Autodesk Inventor part; units mm, degrees
ref_plane "YZ Plane" through (0, 0, 0) normal (1, 0, 0) x (0, 1, 0)
ref_plane "XZ Plane" through (0, 0, 0) normal (0, 1, 0) x (-1, 0, 0)
ref_plane "XY Plane" through (0, 0, 0) normal (0, 0, 1) x (1, 0, 0)
sketch "Sketch1" plane through (0, 0, 0) normal (0, 1, 0) x (-1, 0, 0)
  arc A0 (3.2, -5.2536) -> (17, 0) centre (9.1, 0) ccw
  line L0 (3.2, -5.2536) -> (3.2, -15)
  line L1 (3.2, -15) -> (0, -15)
  line L2 (0, -15) -> (0, 15)
  line L3 (0, 15) -> (3.2, 15)
  line L4 (3.2, 15) -> (3.2, 5.2536)
  arc A1 (17, 0) -> (3.2, 5.2536) centre (9.1, 0) ccw
  line L5 (9.1, 7.9) -> (9.1, -7.9) construction
  line L6 (3.2, 5.2536) -> (17, 0) construction
  line L7 (3.2, -5.2536) -> (17, 0) construction
  point P0 (0, 0)
  point P1 (0, 0)
  dimension "d0" = 3.2
  dimension "d1" = 30
  dimension "d5" = 15.8
  dimension "d6" = 17
extrude "Extrusion1" add sketch "Sketch1" along normal blind 51
sketch "Sketch2" plane through (0, 0, 15) normal (1, 0, 0) x (0, 0, -1)
  circle A0 centre (25.7, 45.35) radius 1.65
  circle A1 centre (4.3, 5.65) radius 1.65
  line L0 (25.7, 45.35) -> (25.7, 5.65) construction
  line L1 (25.7, 5.65) -> (4.3, 5.65) construction
  line L2 (30, 0) -> (30, 51)
  line L3 (0, 0) -> (0, 51)
  line L4 (25.7, 45.35) -> (30, 45.35) construction
  line L5 (25.7, 45.35) -> (30, 51) construction
  line L6 (0, 0) -> (4.3, 5.65) construction
  line L7 (4.3, 5.65) -> (0, 5.65) construction
  line L8 (30, 39.7) -> (22.9, 39.7)
  line L9 (22.9, 39.7) -> (22.9, 0)
  line L10 (22.9, 0) -> (30, 0)
  line L11 (0, 11.3) -> (7.1, 11.3)
  line L12 (7.1, 11.3) -> (7.1, 51)
  line L13 (7.1, 51) -> (0, 51)
  line L14 (25.7, 45.35) -> (30, 39.7) construction
  point P0 (15, 0)
  dimension "d9" = 21.4
  dimension "d10" = 39.7
  dimension "d11" = 3.3
  dimension "d12" = 2.8
extrude "Extrusion2" cut sketch "Sketch2" against normal up to surface (3.2 mm away)
sketch "Sketch3" plane through (0, 0, 0) normal (0, -1, 0) x (1, 0, 0)
  arc A0 (-3.2, 5.2536) -> (-3.2, -5.2536) centre (-9.1, 0) ccw
  circle A1 centre (-9.1, 0) radius 1.5875
  point P0 (0, 0)
  dimension "d15" = 3.175
extrude "Extrusion3" add sketch "Sketch3" along normal blind 11
sketch "Sketch4" plane through (0, 51, 0) normal (0, 1, 0) x (1, 0, 0)
  arc A0 (-3.2, 5.2536) -> (-3.2, -5.2536) centre (-9.1, 0) ccw construction
  circle A1 centre (-9.1, 0) radius 1.5875
  point P0 (0, 0)
  dimension "d18" = 3.175
extrude "Extrusion4" add sketch "Sketch4" along normal blind 11
properties part number "Power Resistor - HSA50" material "Gold"
Could you check a few things on this model? Use its own coordinates, in mm. A direction names the side the tool comes from. Give positions to 0.01 mm unless a question says otherwise; leave off trailing zeros. Loops run counter-clockwise (first coordinate to the right, second up) from the corner with the lowest first, then second, coordinate; pieces in that order, holes last. Notation, with made-up numbers: (14.5, 69.5) -> (68.5, 69.5) arc R17 cw to (68.5, 89.5) -> close; hole circle Ø11 at (-31.75, 71.5). An arc over 180 degrees is marked (long way). Put each result on its own line as item: value.
(1) Please list where these lines run through material, in increasing order: probe 1 along Y at (x, z) = (-2.5, 10.7); probe 2 along Y at (x, z) = (-2.4, -10.7); probe 3 along X at (y, z) = (31.5, -6.5). Write a range as [from, to].
Computed:
probe 1: [0, 4], [7.3, 11.3]
probe 2: [39.7, 43.7], [47, 51]
probe 3: [-13.59, -4.61], [-3.2, 0]
(2) Imagine slicing it at A-A on y = 5.65. Write out the boundary of the cut face in (x, z), plus the area to 3 significant figures.
Computed:
outline: (-17, 0) arc R7.9 ccw to (-3.2, -5.25) -> (-3.2, -7.9) -> (0, -7.9) -> (0, 9.05) -> (-3.2, 9.05) -> (-3.2, 5.25) arc R7.9 ccw to start; (-3.2, 12.35) -> (0, 12.35) -> (0, 15) -> (-3.2, 15) -> close
area: 244 mm^2
(3) I'm going to push flat-ended pins straight in: pin 1 Ø10 at (y, z) = (9, -8) entering from -X; pin 2 Ø1 at (x, y) = (-2.5, 21.5) entering from -Z; pin 3 Ø1.6 at (x, z) = (-1, 13) entering from +Y. Where does each tip first touch, or does it pass through?
Computed:
pin 1: x = -16.41
pin 2: z = -7.9
pin 3: y = 11.3
(4) Imagine slicing it at B-B on z = 10.7. Write out the boundary of the cut face in (x, y), plus the area to 3 significant figures.
Computed:
outline: (-3.2, 0) -> (0, 0) -> (0, 4) -> (-3.2, 4) -> close; (-3.2, 7.3) -> (0, 7.3) -> (0, 11.3) -> (-3.2, 11.3) -> close
area: 25.6 mm^2
(5) For faces 1 (the face through (-10.686, -5.423, -0.07)), 2 (the face through (-2, 11.3, 11)), 3 (the face through (0, 25, 0)), which set-ups out of +Z, -Z, +X, -X, +Y, -Y let a thin tool reach every point of the face, with its end or its side?
Computed:
face 1: -Y
face 2: +Z, +X, -X, +Y
face 3: +Z, -Z, +X, +Y, -Y
(6) Thinking about a two-plate mould opening in X: for faces 4 (the face through (-12.035, 25.143, -7.335)), 5 (the face through (-10.686, 56.423, 0.07)), 6 (the face through (-2, 39.7, -11)), 7 (the face through (-11.79, 25.14, 7.43)), which applies, pulls with the +X half, pulls with the -X half, needs draft (parallel to the pull), parting line crosses it, or undercut?
Computed:
face 4: undercut
face 5: parting line crosses it
face 6: needs draft
face 7: undercut
(7) Imagine slicing it at C-C on x = -9.1. Write out the boundary of the cut face in (y, z), plus the area to 3 significant figures.
Computed:
outline: (-11, -1.59) -> (0, -1.59) -> (0, -7.9) -> (51, -7.9) -> (51, -1.59) -> (62, -1.59) -> (62, 1.59) -> (51, 1.59) -> (51, 7.9) -> (0, 7.9) -> (0, 1.59) -> (-11, 1.59) -> close
area: 876 mm^2
(8) Imagine slicing it at D-D on y = 36. Write out the boundary of the cut face in (x, z), plus the area to 3 significant figures.
Computed:
outline: (-17, 0) arc R7.9 ccw to (-3.2, -5.25) -> (-3.2, -7.9) -> (0, -7.9) -> (0, 7.9) -> (-3.2, 7.9) -> (-3.2, 5.25) arc R7.9 ccw to start
area: 232 mm^2
